Could you check a few things on this model? Use its own coordinates, in mm. A direction names the side the tool comes from. Round coordinates to 2 decimals unless told otherwise and drop trailing zeros. Write each loop counter-clockwise with the first axis right and the second up, starting at its lowest first coordinate (ties: lowest second). Pieces come first, ordered by that corner, then holes. Notation, with made-up numbers: (73.5, -28) -> (118.5, -28) arc R8 cw to (118.5, -19) -> close; hole circle Ø9 at (74.5, 20.25). An arc over 180 degrees is marked (long way). Return JSON: item names as keys, results as strings.
from build123d import *

# Parameters (mm, degrees)
F1_W        = 100
F1_H        = 100
F2_DEPTH    = 2.5
F4_W        = 95
F4_H        = 95
F5_DEPTH    = 2.5
F7_W        = 45
F7_H        = 45
F8_DEPTH    = 75
F9_T        = 2.5
F9_T3_DEPTH = 100
F9_T5_DEPTH = 100
F9_T7_DEPTH = 50
F9_T9_DEPTH = 50


# Not quite as in the source:
# - a shell that OpenCascade refuses in one call is made with other operations: the cavity is built on its own and cut out


with BuildPart() as f2:
    # F1 (on offset) → F2 (new body)
    with BuildSketch(Plane.XY.offset(80)):
        Rectangle(F1_W, F1_H)
    extrude(amount=-F2_DEPTH)

    # F4 (on offset) → F5 (join)
    with BuildSketch(Plane.XY.offset(77.5)):
        Rectangle(F4_W, F4_H)
    extrude(amount=-F5_DEPTH)

    # F7 (on offset) → F8 (join)
    with BuildSketch(Plane.XY.offset(75)):
        Rectangle(F7_W, F7_H)
    extrude(amount=-F8_DEPTH)

    # F9: shell of thickness 2.5, made by hand


with BuildPart() as f9_core1:
    # F9_t2: copy of F2
    add(f2.part)

    # the walls: a layer under each face that stays
    f9_faces = [f9_core1.faces().sort_by_distance(p)[0] for p in [
        (0, 50, 78.75),
        (50, 0, 78.75),
        (-50, 0, 78.75),
        (34.375, -48.7654320988, 77.5),
        (0, -50, 78.75),
        (-47.5, 0, 76.25),
        (0, -47.5, 76.25),
        (47.5, 0, 76.25),
        (0, 47.5, 76.25),
        (-31.6666666667, -31.6666666667, 75),
        (-22.5, 0, 37.5),
        (0, -22.5, 37.5),
        (22.5, 0, 37.5),
        (0, 22.5, 37.5),
        (0, 0, 0),
    ]]
    thicken(f9_faces, amount=-F9_T, mode=Mode.SUBTRACT)

    # F9_s4 → F9_t3 (cut)
    with BuildSketch(Plane.XZ.offset(-50)):
        Polygon((-47.525, 77.475), (-47.5, 80), (-45, 80), (-45, 77.5), align=None)
        Polygon((47.525, 77.475), (47.5, 80), (45, 80), (45, 77.5), align=None)
    extrude(amount=F9_T3_DEPTH, mode=Mode.SUBTRACT)

    # F9_s6 → F9_t5 (cut)
    with BuildSketch(Plane.YZ.offset(-50)):
        Polygon((-47.525, 77.475), (-47.5, 80), (-45, 80), (-45, 77.5), align=None)
        Polygon((47.525, 77.475), (47.5, 80), (45, 80), (45, 77.5), align=None)
    extrude(amount=F9_T5_DEPTH, mode=Mode.SUBTRACT)

    # F9_s8 → F9_t7 (cut)
    with BuildSketch(Plane.XZ.offset(-25)):
        Polygon((-22.525, 74.975), (-22.5, 77.5), (-20, 77.5), (-20, 75), align=None)
        Polygon((22.525, 74.975), (22.5, 77.5), (20, 77.5), (20, 75), align=None)
    extrude(amount=F9_T7_DEPTH, mode=Mode.SUBTRACT)

    # F9_s10 → F9_t9 (cut)
    with BuildSketch(Plane.YZ.offset(-25)):
        Polygon((-22.525, 74.975), (-22.5, 77.5), (-20, 77.5), (-20, 75), align=None)
        Polygon((22.525, 74.975), (22.5, 77.5), (20, 77.5), (20, 75), align=None)
    extrude(amount=F9_T9_DEPTH, mode=Mode.SUBTRACT)


with BuildPart() as f2_1:
    add(f2.part)

    # what is left inside the walls is the cavity
    f9_cavity = [f9_core1.part.solids().sort_by_distance(p)[0] for p in [
        (0, -15, 79.975),
    ]]
    add(f9_cavity, mode=Mode.SUBTRACT)


solid = f2_1.part
1) Thinking about a two-plate mould opening in X: for faces 1 (the face through (-1, -50, 79)), 2 (the face through (1, 21, 77.5)), 3 (the face through (0, 20, 41)), 4 (the face through (22.5, 0, 38)), which applies, pulls with the +X half, pulls with the -X half, needs draft (parallel to the pull), parting line crosses it, or undercut?
Return value:
{"face 1": "needs draft", "face 2": "undercut", "face 3": "undercut", "face 4": "pulls with the +X half"}
2) I want a section at A-A, the plane z = 49. Please give me the cut outline in (x, y), and give its area (3 significant figures).
Return value:
{"outline": "(-22.5, -22.5) -> (22.5, -22.5) -> (22.5, 22.5) -> (-22.5, 22.5) -> close; hole (-20, -20) -> (20, -20) -> (20, 20) -> (-20, 20) -> close", "area": "425 mm²"}
3) For faces 5 (the face through (-20, 0, 41)), 6 (the face through (47.5, -1, 76)), 7 (the face through (-47.5, -1, 76)), 8 (the face through (0, 22.5, 38)), which set-ups out of +Z, -Z, +X, -X, +Y, -Y let a thin tool reach every point of the face, with its end or its side?
Return value:
{"face 5": "+Z", "face 6": "-Z, +X, +Y, -Y", "face 7": "-Z, -X, +Y, -Y", "face 8": "-Z, +X, -X, +Y"}
4) I want a section at D-D, the plane x = -1.5. Please give me the cut outline in (y, z).
Return value:
{"outline": "(-50, 77.5) -> (-47.5, 77.5) -> (-47.5, 75) -> (-22.5, 75) -> (-22.5, 0) -> (22.5, 0) -> (22.5, 75) -> (47.5, 75) -> (47.5, 77.5) -> (50, 77.5) -> (50, 80) -> (45, 80) -> (45, 77.5) -> (20, 77.5) -> (20, 2.5) -> (-20, 2.5) -> (-20, 77.5) -> (-45, 77.5) -> (-45, 80) -> (-50, 80) -> close"}
5) If I drill on probe 1 along X at (y, z) = (12, 12.5); probe 2 along Y at (x, z) = (12, 76.5), over which ranges is the centre line in solid material (lowest first)? Write a range as [from, to].
Return value:
{"probe 1": "[-22.5, -20], [20, 22.5]", "probe 2": "[-47.5, -20], [20, 47.5]"}
6) Will these pins go through, and if not, where does the flat tip stop? pin 1 Ø8 at (y, z) = (-6.5, 14.5) entering from -X; pin 2 Ø12 at (x, y) = (-5, -2.5) entering from +Z; pin 3 Ø5 at (x, z) = (-26, 27.5) entering from +Y; pin 4 Ø4 at (x, z) = (-14.5, 69) entering from -Y.
Return value:
{"pin 1": "x = -22.5", "pin 2": "z = 2.5", "pin 3": "through", "pin 4": "y = -22.5"}
7) I want a section at B-B, the plane x = -40. Please give me the cut outline in (y, z), and give its area (4 significant figures).
Return value:
{"outline": "(-50, 77.5) -> (-47.5, 77.5) -> (-47.5, 75) -> (47.5, 75) -> (47.5, 77.5) -> (50, 77.5) -> (50, 80) -> (45, 80) -> (45, 77.5) -> (-45, 77.5) -> (-45, 80) -> (-50, 80) -> close", "area": "262.5 mm²"}
